Can you work these out from the model? Positions are in its coordinate system, mm. Face numbers are marked on the shaded views. A direction names the side the tool comes from. Coordinates: 2 decimals unless noted, no trailing zeros. Order: outer loops, then holes, each group sorted by start corner. A loop starts at its lowest first (then second) coordinate and runs counter-clockwise, first axis right, second up. Notation, with made-up numbers: (80.25, 34) -> (99.25, 34) arc R24 cw to (99.25, 70) -> close; hole circle Ø10 at (4, 49). An arc over 180 degrees is marked (long way). Answer in a Markdown table with one row per item. Add a question column.
1. On a 3-axis mill with a long thin cutter (end or side, diameter ignored), from which of +Z, -Z, +X, -X, +Y, -Y can I reach the whole of each face in a straight line? I mean the marked faces 4, 5, 6, 7 and 8. Say none if no direction works.
2. Imagine slicing it at C-C on z = -0.5. Write out the boundary of the cut face in (x, y).
3. If I drill on line 1 along X through (y, z) = (7.5, -3); line 2 along Z through (x, y) = (-30.5, 14.5); line 3 along Z through (x, y) = (19.05, 0.8), over which ranges is the centre line in solid material (lowest first)? Write a range as [from, to].
4. Will these pins go through, and if not, where does the flat tip stop? pin 1 (2.5 mm diameter, centred on y = 20, z = 9, fed in from -X); pin 2 (1.8 mm diameter, centred on x = 19.05, z = 10, fed in from -Y); pin 3 (13.5 mm diameter, centred on x = 6, y = 7.5, fed in from +Z); pin 4 (2.5 mm diameter, centred on x = 18, z = 12, fed in from +Y).
5. Imagine slicing it at B-B on x = 19.05. Write out the boundary of the cut face in (y, z).
6. Imagine slicing it at D-D on x = 11.5. Write out the boundary of the cut face in (y, z), plus the area to 3 significant figures.
7. We'd pull the mould along X, two halves only. Please class the marked faces 1, 2 and 3: pulls with the +X half, pulls with the -X half, needs draft (parallel to the pull), parting line crosses it, or undercut.
8. Imagine slicing it at A-A on z = 10. Write out the boundary of the cut face in (x, y).
from build123d import *

# Parameters (mm, degrees)
SKETCH1_W           = 69.977
SKETCH1_H           = 11
BOSS_EXTRUDE1_DEPTH = 2
BOSS_EXTRUDE2_START = 2
SKETCH1_4_W         = 3.175
SKETCH1_4_H         = 3
BOSS_EXTRUDE2_DEPTH = 25.4
SKETCH3_W           = 9
SKETCH3_H           = 9
SKETCH3_R           = 1.5
BOSS_EXTRUDE3_DEPTH = 2
BOSS_EXTRUDE4_DEPTH = 2
BOSS_EXTRUDE5_START = -47.1
BOSS_EXTRUDE5_DEPTH = 2


with BuildPart() as part:
    # Sketch1 → Boss-Extrude1 (new body)
    with BuildSketch(Plane(origin=(0, 0, 0), x_dir=(1, 0, 0), z_dir=(0, 1, 0))):
        Rectangle(SKETCH1_W, SKETCH1_H)
    extrude(amount=BOSS_EXTRUDE1_DEPTH)

    # Sketch1<4> → Boss-Extrude2 (add)
    with BuildSketch(Plane(origin=(0, 0, 0), x_dir=(1, 0, 0), z_dir=(0, 1, 0)).offset(BOSS_EXTRUDE2_START)):
        Polygon((34.9885, -5.5), (34.9885, -0.5), (31.8135, -0.5), (-31.8135, -0.5), (-34.9885, -0.5), (-34.9885, -5.5), align=None)
        Polygon((-6.477, 2.5), (-6.477, 5.5), (-34.9885, 5.5), (-34.9885, 2.5), (-31.8135, 2.5), align=None)
        Polygon((34.9885, 2.5), (34.9885, 5.5), (6.477, 5.5), (6.477, 2.5), (31.8135, 2.5), align=None)
        with Locations((-33.401, 1)):
            Rectangle(SKETCH1_4_W, SKETCH1_4_H)
        with Locations((33.401, 1)):
            Rectangle(SKETCH1_4_W, SKETCH1_4_H)
    extrude(amount=BOSS_EXTRUDE2_DEPTH)

    # Sketch3 → Boss-Extrude3 (add)
    with BuildSketch(Plane.XZ):
        with Locations((-19.05, 10)):
            Rectangle(SKETCH3_W, SKETCH3_H)
        with Locations((-19.05, 10)):
            Circle(SKETCH3_R, mode=Mode.SUBTRACT)
        with Locations((19.05, 10)):
            Rectangle(SKETCH3_W, SKETCH3_H)
        with Locations((19.05, 10)):
            Circle(SKETCH3_R, mode=Mode.SUBTRACT)
    extrude(amount=-BOSS_EXTRUDE3_DEPTH)

    # Sketch4 → Boss-Extrude4 (add)
    with BuildSketch(Plane.ZY.offset(23.55)):
        Polygon((14.5, 0), (5.5, 27.4), (5.5, 0), align=None)
    extrude(amount=BOSS_EXTRUDE4_DEPTH)

    # Sketch4<2> → Boss-Extrude5 (add)
    with BuildSketch(Plane.ZY.offset(23.55).offset(BOSS_EXTRUDE5_START)):
        Polygon((14.5, 0), (5.5, 27.4), (5.5, 0), align=None)
    extrude(amount=-BOSS_EXTRUDE5_DEPTH)


solid = part.part
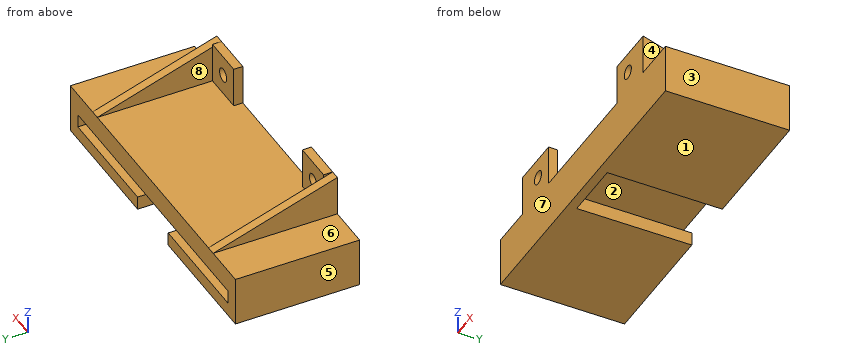
Answers follow:
| question | item | result |
|---|---|---|
| 1 | face 4 | +Z, +X, +Y, -Y |
| 1 | face 5 | +Z, -Z, -X, +Y, -Y |
| 1 | face 6 | +Z, -X, +Y, -Y |
| 1 | face 7 | +Z, -Z, +X, -X, -Y |
| 1 | face 8 | +Z, +Y |
| 2 | outline | (-34.99, 0) -> (34.99, 0) -> (34.99, 27.4) -> (31.81, 27.4) -> (31.81, 2) -> (-31.81, 2) -> (-31.81, 27.4) -> (-34.99, 27.4) -> close |
| 3 | line 1 | x = [-34.99, -6.48], [6.48, 34.99] |
| 3 | line 2 | z = [-5.5, -2.5], [0.5, 5.5] |
| 3 | line 3 | z = [-5.5, 8.5], [11.5, 14.5] |
| 4 | pin 1 | stops at x = -25.55 |
| 4 | pin 2 | passes through |
| 4 | pin 3 | stops at z = 5.5 |
| 4 | pin 4 | stops at y = 2 |
| 5 | outline | (0, -5.5) -> (27.4, -5.5) -> (27.4, -2.5) -> (2, -2.5) -> (2, 0.5) -> (27.4, 0.5) -> (27.4, 5.5) -> (2, 5.5) -> (2, 8.5) -> (0, 8.5) -> close; (0, 11.5) -> (2, 11.5) -> (2, 14.5) -> (0, 14.5) -> close |
| 6 | outline | (0, -5.5) -> (27.4, -5.5) -> (27.4, -2.5) -> (2, -2.5) -> (2, 0.5) -> (27.4, 0.5) -> (27.4, 5.5) -> (0, 5.5) -> close |
| 6 | area | 225 mm² |
| 7 | face 1 | needs draft |
| 7 | face 2 | undercut |
| 7 | face 3 | pulls with the +X half |
| 8 | outline | (-25.55, 0) -> (-20.55, 0) -> (-20.55, 2) -> (-23.55, 2) -> (-23.55, 13.7) -> (-25.55, 13.7) -> close; (-17.55, 0) -> (-14.55, 0) -> (-14.55, 2) -> (-17.55, 2) -> close; (14.55, 0) -> (17.55, 0) -> (17.55, 2) -> (14.55, 2) -> close; (20.55, 0) -> (25.55, 0) -> (25.55, 13.7) -> (23.55, 13.7) -> (23.55, 2) -> (20.55, 2) -> close |
